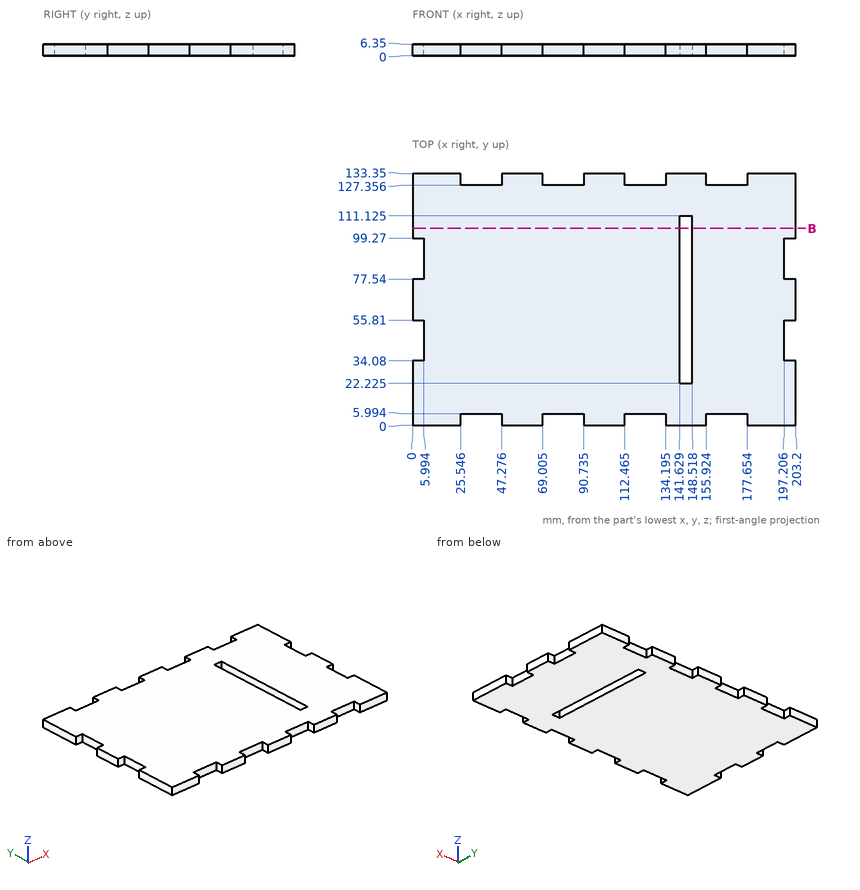
Geometry check sheet. Reference: drawing and pictorial views, mm from the part's lowest x, y, z. Round coordinates to 2 decimals unless told otherwise and drop trailing zeros. Loops run counter-clockwise (first coordinate to the right, second up) from the corner with the lowest first, then second, coordinate; pieces in that order, holes last. Notation, with made-up numbers: (47.25, -25) - (94.25, -25) arc R14 ccw to (94.25, 1) - close; hole circle Ø10 at (44, -33). An arc over 180 degrees is marked (long way). Write item = value, one per line. Start each with the question number.
Q1. Section check B-B (y = 104.5). Record the boundary of the cut face in (x, z), plus the area to 3 significant figures.
Q2. Thickness scan on L1, parallel to X at y = 39.5, z = 5.75 (1 decimal); L2, parallel to X at y = 59, z = 4.75; L3, parallel to Y at x = 82, z = 5.75 (1 decimal). Record the ranges inside material, lowest first.
Q3. Depth check by flat-ended pin: P1, Ø3, axis at x = 38.5, z = 2, coming from the +Y side; P2, Ø2, axis at y = 50.5, z = 4.5, coming from the +X side. Enter the tip coordinate at first touch or a pass-through.
Derived:
q1.outline = (0, 0) - (141.63, 0) - (141.63, 6.35) - (0, 6.35) - close; (148.52, 0) - (203.2, 0) - (203.2, 6.35) - (148.52, 6.35) - close
q1.area = 1,250 mm^2
q2.L1 = 6 to 141.6, 148.5 to 197.2
q2.L2 = 0 to 141.63, 148.52 to 203.2
q2.L3 = 6 to 127.4
q3.P1 = 127.36
q3.P2 = 197.21
